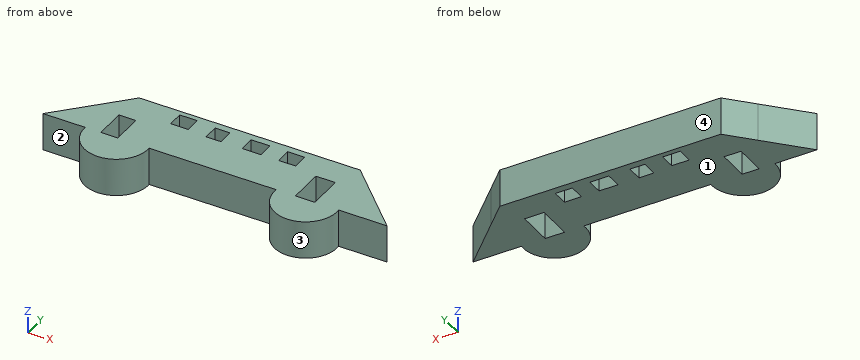
```python
from build123d import *

# Parameters (mm, degrees)
F0_W     = 7.7999122441
F0_H     = 6.8999230862
F0_W_2   = 6.5999259241
F0_W_3   = 8.3999030758
F0_W_4   = 7.4999127537
F0_W_5   = 17.3998039681
F0_H_2   = 13.469719328
F0_W_6   = 19.7997752111
F1_DEPTH = 16.764


with BuildPart() as f1:
    # F0 (on Top) → F1 (new body)
    with BuildSketch(Plane.XY):
        with BuildLine():
            Line((-59.4818092616, 16.9173511698), (-75.65433532, 0))
            Line((-75.65433532, 0), (-56.9691322744, 0))
            Line((-56.9691322744, 0), (-50.0688962638, 0))
            Line((-50.0688962638, 0), (-50.0688962638, 13.7697160244))
            Line((-50.0688962638, 13.7697160244), (-42.5689779222, 13.7697160244))
            Line((-42.5689779222, 13.7697160244), (-42.5689779222, 0))
            Line((-42.5689779222, 0), (-30.2691180259, 0))
            Line((-30.2691180259, 0), (-30.2691180259, 13.469719328))
            Line((-30.2691180259, 13.469719328), (-14.36929591, 13.469719328))
            Line((-14.36929591, 13.469719328), (3.0305080581, 13.469719328))
            Line((3.0305080581, 13.469719328), (22.8302832693, 13.469719328))
            Line((22.8302832693, 13.469719328), (22.8302832693, 0))
            Line((22.8302832693, 0), (27.537882328, 0))
            Line((27.537882328, 0), (36.0301360488, 0))
            Line((36.0301360488, 0), (36.0301360488, 15.5696962029))
            Line((36.0301360488, 15.5696962029), (44.6445176616, 15.5696962029))
            Line((44.6445176616, 15.5696962029), (44.6445176616, 0))
            Line((44.6445176616, 0), (55.1420748234, 0))
            Line((55.1420748234, 0), (76.5484273434, 0))
            Line((76.5484273434, 0), (57.7259496837, 18.6665190633))
            ThreePointArc((57.7259496837, 18.6665190633), (44.6445176616, 18.7276304562), (35.1301468909, 27.7056228369))
            Line((35.1301468909, 27.7056228369), (-36.2690500915, 27.7056228369))
            ThreePointArc((-36.2690500915, 27.7056228369), (-46.0901653841, 18.4701942224), (-59.4818092616, 16.9173511698))
        make_face()
        with Locations((-26.0691642761, 22.0196228474)):
            Rectangle(F0_W, F0_H, mode=Mode.SUBTRACT)
        with Locations((-10.4693404865, 21.1196336895)):
            Rectangle(F0_W_2, F0_H, mode=Mode.SUBTRACT)
        with Locations((6.3304699725, 21.1196336895)):
            Rectangle(F0_W_3, F0_H, mode=Mode.SUBTRACT)
        with Locations((22.0802919939, 21.1196336895)):
            Rectangle(F0_W_4, F0_H, mode=Mode.SUBTRACT)
        with BuildLine():
            Line((-49.1685159504, 27.7056228369), (-59.4818092616, 16.9173511698))
            ThreePointArc((-59.4818092616, 16.9173511698), (-46.0901653841, 18.4701942224), (-36.2690500915, 27.7056228369))
            Line((-36.2690500915, 27.7056228369), (-49.1685159504, 27.7056228369))
        make_face()
        with BuildLine():
            Line((48.6113242805, 27.7056228369), (35.1301468909, 27.7056228369))
            ThreePointArc((35.1301468909, 27.7056228369), (44.6445176616, 18.7276304562), (57.7259496837, 18.6665190633))
            Line((57.7259496837, 18.6665190633), (48.6113242805, 27.7056228369))
        make_face()
        with Locations((-5.6693939259, 6.734859664)):
            Rectangle(F0_W_5, F0_H_2)
        with Locations((12.9303956637, 6.734859664)):
            Rectangle(F0_W_6, F0_H_2)
        Polygon((-30.2691180259, 0), (-28.6692157388, 0), (-14.36929591, 0), (-14.36929591, 13.469719328), (-30.2691180259, 13.469719328), align=None)
        with BuildLine():
            ThreePointArc((27.537882328, 0), (41.3399785757, -15.2172739199), (55.1420748234, 0))
            Line((55.1420748234, 0), (44.6445176616, 0))
            Line((44.6445176616, 0), (36.0301360488, 0))
            Line((36.0301360488, 0), (27.537882328, 0))
        make_face()
        with BuildLine():
            Line((-50.0688962638, 0), (-56.9691322744, 0))
            ThreePointArc((-56.9691322744, 0), (-42.8191740066, -14.7643966846), (-28.6692157388, 0))
            Line((-28.6692157388, 0), (-30.2691180259, 0))
            Line((-30.2691180259, 0), (-42.5689779222, 0))
            Line((-42.5689779222, 0), (-50.0688962638, 0))
        make_face()
    extrude(amount=-F1_DEPTH)


solid = f1.part
```
Geometry check sheet. Reference: the model listing, model coordinates, mm. Face numbers are marked on the shaded views. A direction names the side the tool comes from. Round coordinates to 2 decimals unless told otherwise and drop trailing zeros. Loops run counter-clockwise (first coordinate to the right, second up) from the corner with the lowest first, then second, coordinate; pieces in that order, holes last. Notation, with made-up numbers: M -12.5,16.5 L 5.5,16.5 A23 ccw 5.5,53.5 Z; hole C 13.25,75.25 d5. An arc over 180 degrees is marked long. Return JSON: item names as keys, results as strings. Group by question number.
(1) Scan lines: line 1 along Y through (x, z) = (41, -12.25); line 2 along Y through (x, z) = (22, -2.25); line 3 along X through (y, z) = (19.5, -0.75). Record each from-to range of solid material in increasing order. Write a range as [from, to].
(2) Section check A-A, the plane z = -6.5. Give the number of separate pieces and of enclosed holes in the cut face, and give its area (3 significant figures).
(3) Section check C-C, the plane x = 21. Enter the section's corners in (y, z).
(4) Section check B-B, the plane y = 2. Enter the section's corners in (x, z), and give its area (3 significant figures).
(5) Go/stop test with flat-tipped pins: pin 1 (8 mm diameter, centred on y = -7, z = -3, fed in from +X); pin 2 (6.5 mm diameter, centred on x = 8, z = -11.5, fed in from -Y); pin 3 (6 mm diameter, centred on x = -29, y = -3, fed in from +Z); pin 4 (3 mm diameter, centred on y = 11.5, z = -12.5, fed in from +X). Record where each tip stops, or that it passes through.
(6) Section check D-D, the plane y = -8.5. Enter the section's corners in (x, z) (3 decimals).
(7) Set-up check for the marked faces 1 and 2: record each of +Z, -Z, +X, -X, +Y, -Y from which the full face is reachable in a straight line by a thin tool's end or side.
(8) Mould release check, pull along X, two halves, no side actions. Record for the marked faces 3 and 4: pulls with the +X half, pulls with the -X half, needs draft (parallel to the pull), parting line crosses it, or undercut.
Data:
{
 "1": {"line 1": "[-15.21, 0], [15.57, 27.71]", "line 2": "[0, 17.67], [24.57, 27.71]", "line 3": "[-57.01, -29.97], [-22.17, -13.77], [-7.17, 2.13], [10.53, 18.33], [25.83, 56.89]"},
 "2": {"separate pieces": "1", "enclosed holes": "6", "area": "3,690 mm²"},
 "3": {"outline": "M 0,-16.76 L 17.67,-16.76 L 17.67,0 L 0,0 Z; M 24.57,-16.76 L 27.71,-16.76 L 27.71,0 L 24.57,0 Z"},
 "4": {"outline": "M -73.74,-16.76 L -50.07,-16.76 L -50.07,0 L -73.74,0 Z; M -42.57,-16.76 L 36.03,-16.76 L 36.03,0 L -42.57,0 Z; M 44.64,-16.76 L 74.53,-16.76 L 74.53,0 L 44.64,0 Z", "area": "2,220 mm²"},
 "5": {"pin 1": "x = 55.11", "pin 2": "y = 0", "pin 3": "z = 0", "pin 4": "x = 66.46"},
 "6": {"outline": "M -54.575,-16.764 L -31.063,-16.764 L -31.063,0 L -54.575,0 Z; M 29.458,-16.764 L 53.222,-16.764 L 53.222,0 L 29.458,0 Z"},
 "7": {"face 1": "-Z, +X, -X, +Y, -Y", "face 2": "+Z, -Z, -X, -Y"},
 "8": {"face 3": "undercut", "face 4": "needs draft"}
}
